Read the model definition and answer for the solid it produces. Units are mm, in the model's axes. A direction names the side the tool comes from. Coordinates: 2 decimals unless noted, no trailing zeros. Order: outer loops, then holes, each group sorted by start corner. A loop starts at its lowest first (then second) coordinate and runs counter-clockwise, first axis right, second up. Notation, with made-up numbers: M 35.5,-7 L 47.5,-7 A21 cw 47.5,20 Z; hole C -10.75,82 d11. An arc over 180 degrees is marked long. Use a Markdown table: item, result. Add a question column.
1) For faces 4 (the face through (139.239, 126, 297)), 5 (the face through (109.71, 31.48, 333.61)), 6 (the face through (119.62, -139.58, 328.38)), determine the directions among +Z, -Z, +X, -X, +Y, -Y from which every point of the face is accessible in a straight line to the end or side of a thin tool.
2) The mould has two halves that part along Z. Classify faces 1 (the face through (113, -95, 660.4)), 2 (the face through (48.316, -60.083, 553.686)), 3 (the face through (150.18, -84.39, 290.84)): released by +Z, released by -Z, zero draft, split by the parting line, or undercut.
3) Find the intervals of material crossed by probe 1 along X at (y, z) = (0, 393.5); probe 2 along X at (y, z) = (0, 518); probe 3 along Z at (x, y) = (112.5, 0), in increasing order. Write a range as [from, to].
4) Each of these flat-tipped pins is pushed along its axis until it touches: pin 1 Ø8 at (x, z) = (93.5, 272.5) entering from +Y; pin 2 Ø12 at (y, z) = (-52, 331) entering from -X; pin 3 Ø2 at (x, y) = (200, -6.5) entering from +Z. Where does it stop, or does it pass through?
5) Find section D-D on z = 279.4. Write down the section's boundary in (x, y), plus the area to 3 significant figures.
6) Find section C-C on z = 14. Write down the section's boundary in (x, y).
7) Find section B-B on y = -60.5. Count the separate pieces of the cut face and the enclosed holes in it, plus the area to 3 significant figures.
8) Find section A-A on z = 183.5. Write down the section's boundary in (x, y), plus the area to 3 significant figures.
from build123d import *

# Parameters (mm, degrees)
F2_SIZE   = 5.08
F4_DEPTH  = 806.27653
F6_R      = 76.2
F7_DEPTH  = 635.34323
F8_R      = 31.75
F9_DEPTH  = 343.56878
F10_R     = 38.1
F11_DEPTH = 418.60546


with BuildPart() as f1:
    # F0 (on Front) → F1 (revolve)
    with BuildSketch(Plane.XZ):
        with BuildLine():
            Line((202.739415619, 454.8578867186), (113.839415619, 454.8578867186))
            Line((113.839415619, 454.8578867186), (113.839415619, -139.7))
            ThreePointArc((113.839415619, -139.7), (212.6222329507, -98.7828173318), (253.539415619, 0))
            Line((253.539415619, 0), (253.539415619, 647.7))
            ThreePointArc((253.539415619, 647.7), (249.81967174, 656.6802561211), (240.839415619, 660.4))
            Line((240.839415619, 660.4), (202.739415619, 660.4))
            Line((202.739415619, 660.4), (202.739415619, 454.8578867186))
        make_face()
    revolve(axis=Axis((113.839415619, 0, 157.5789433593), (0, 0, -1)))

    # F2
    f2_edges = [f1.edges().sort_by_distance(p)[0] for p in [
        (24.939416, 0, 660.4),
    ]]
    chamfer(f2_edges, length=F2_SIZE)

    # F3 (on face) → F4 (cut)
    with BuildSketch(Plane.XY.offset(660.4)):
        with BuildLine():
            Line((139.239415619, 154.6271294355), (88.439415619, 154.6271294355))
            Line((88.439415619, 154.6271294355), (88.439415619, 124.4340789334))
            ThreePointArc((88.439415619, 124.4340789334), (113.839415619, 127), (139.239415619, 124.4340789334))
            Line((139.239415619, 124.4340789334), (139.239415619, 154.6271294355))
        make_face()
        with BuildLine():
            ThreePointArc((139.239415619, 124.4340789334), (113.839415619, 127), (88.439415619, 124.4340789334))
            Line((88.439415619, 124.4340789334), (88.439415619, 114.3))
            Line((88.439415619, 114.3), (139.239415619, 114.3))
            Line((139.239415619, 114.3), (139.239415619, 124.4340789334))
        make_face()
    extrude(amount=-F4_DEPTH, mode=Mode.SUBTRACT)

    # F6 (on offset) → F7 (cut)
    with BuildSketch(Plane.YZ.offset(-152.4)):
        with Locations((0, 139.7)):
            Circle(F6_R)
    extrude(amount=F7_DEPTH, mode=Mode.SUBTRACT)

    # F8 (on face) → F9 (cut)
    with BuildSketch(Plane.XY.offset(454.8578867186)):
        with Locations((113.839415619, 0)):
            Circle(F8_R)
    extrude(amount=-F9_DEPTH, mode=Mode.SUBTRACT)

    # F10 (on Front) → F11 (cut)
    with BuildSketch(Plane.XZ):
        with Locations((113.839415619, 279.4)):
            Circle(F10_R)
    extrude(amount=F11_DEPTH, mode=Mode.SUBTRACT)


solid = f1.part
Check result:
| question | item | result |
|---|---|---|
| 1 | face 4 | +Z, -Z, +Y |
| 1 | face 5 | +Z |
| 1 | face 6 | +Z, -Z |
| 2 | face 1 | released by +Z |
| 2 | face 2 | zero draft |
| 2 | face 3 | undercut |
| 3 | probe 1 | x = [-25.86, 82.09], [145.59, 253.54] |
| 3 | probe 2 | x = [-25.86, 24.94], [202.74, 253.54] |
| 3 | probe 3 | z = [-139.69, 63.5] |
| 4 | pin 1 | stops at y = 114.3 |
| 4 | pin 2 | stops at x = -18.07 |
| 4 | pin 3 | stops at z = 454.86 |
| 5 | outline | M 75.74,-134.4 L 75.74,0 L 82.09,0 A31.75 cw 145.59,0 L 151.94,0 L 151.94,-134.4 A139.7 ccw 139.24,137.37 L 139.24,114.3 L 88.44,114.3 L 88.44,137.37 A139.7 ccw Z |
| 5 | area | 48,000 mm2 |
| 6 | outline | M 88.44,114.3 L 88.44,137.37 A139.7 ccw long 139.24,137.37 L 139.24,114.3 Z |
| 7 | separate pieces | 2 |
| 7 | enclosed holes | 1 |
| 7 | area | 136,000 mm2 |
| 8 | outline | M -11.17,-62.35 A139.7 ccw 238.85,-62.35 Z; M -11.17,62.35 L 238.85,62.35 A139.7 ccw 139.24,137.37 L 139.24,114.3 L 88.44,114.3 L 88.44,137.37 A139.7 ccw Z |
| 8 | area | 26,400 mm2 |
